Verification items for this drawing (mm, ordinates from the low corner). A direction names the side the tool comes from. Round coordinates to 2 decimals unless told otherwise and drop trailing zeros. Order: outer loops, then holes, each group sorted by start corner. A loop starts at its lowest first (then second) coordinate and runs counter-clockwise, first axis right, second up. Notation, with made-up numbers: (78, 59.5) -> (86, 59.5) arc R22 ccw to (86, 87.5) -> close; hole circle Ø10 at (2, 61). An arc over 180 degrees is marked (long way). Put each result on its own line as item: value.
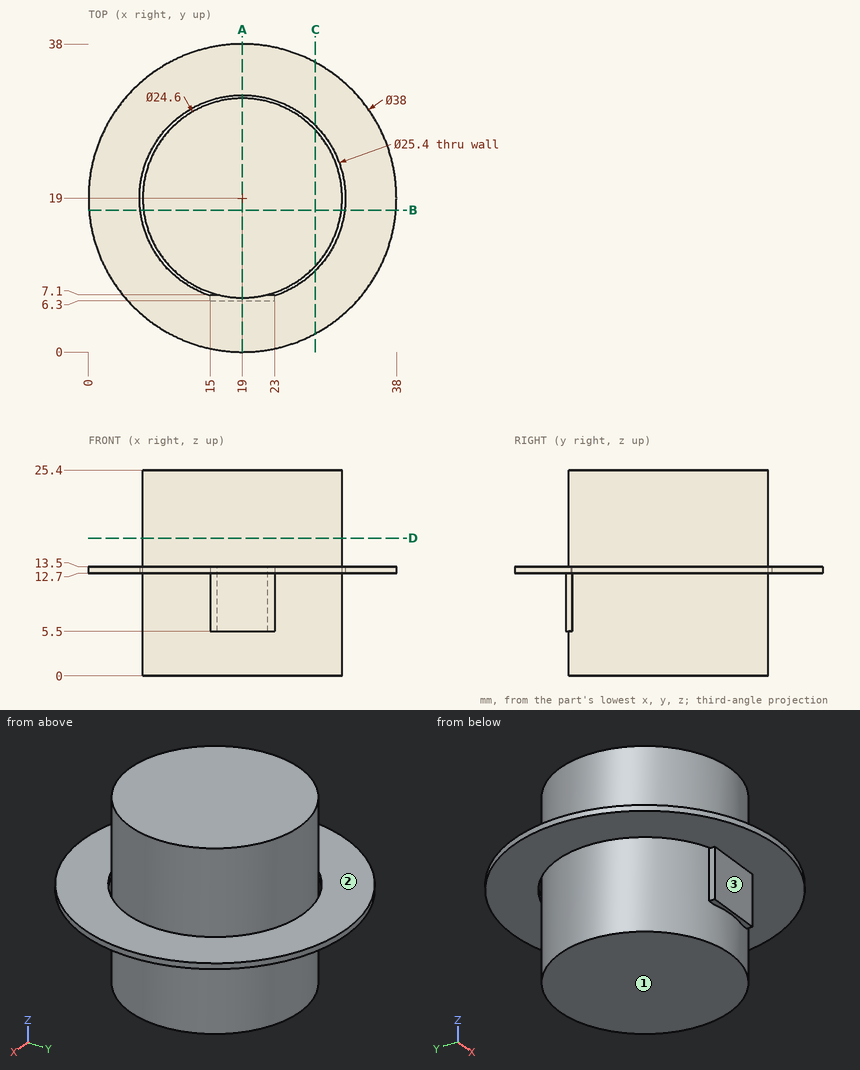
Item 1: Section check D-D on z = 17. Record the boundary of the cut face in (x, y), then the cut area to 3 significant figures.
Check sheet entries:
outline: circle Ø24.6 at (19, 19)
area: 475 mm^2
Item 2: Tool access check on the marked faces 1, 2 and 3. Record the directions out of +Z, -Z, +X, -X, +Y, -Y that give a thin tool (end or side, any length) a straight path to the whole face; none if there is none.
Check sheet entries:
face 1: -Z, +X, -X, +Y, -Y
face 2: +Z
face 3: -Z, +X, -X, -Y
Item 3: Gauge pin test, flat ends, axial feed: pin 1 Ø2 at (x, z) = (11.5, 13) entering from -Y; pin 2 Ø1.5 at (x, z) = (24.5, 22) entering from -Y; pin 3 Ø1.5 at (y, z) = (10.5, 17) entering from -X. Record the tip position at first contact, or that the pin passes through.
Check sheet entries:
pin 1: stops at y = 1.15
pin 2: stops at y = 7.65
pin 3: stops at x = 9.45
Item 4: Section check C-C on x = 28. Record the boundary of the cut face in (y, z), then the cut area to 3 significant figures.
Check sheet entries:
outline: (2.27, 12.7) -> (10.04, 12.7) -> (10.04, 13.5) -> (2.27, 13.5) -> close; (10.62, 0) -> (27.38, 0) -> (27.38, 25.4) -> (10.62, 25.4) -> close; (27.96, 12.7) -> (35.73, 12.7) -> (35.73, 13.5) -> (27.96, 13.5) -> close
area: 438 mm^2
Item 5: Section check A-A on x = 19. Record the boundary of the cut face in (y, z).
Check sheet entries:
outline: (0, 12.7) -> (6.3, 12.7) -> (6.3, 5.5) -> (6.7, 5.5) -> (6.7, 0) -> (31.3, 0) -> (31.3, 25.4) -> (6.7, 25.4) -> (6.7, 13.5) -> (0, 13.5) -> close; (31.7, 12.7) -> (38, 12.7) -> (38, 13.5) -> (31.7, 13.5) -> close
Item 6: Section check B-B on y = 17.5. Record the boundary of the cut face in (x, z).
Check sheet entries:
outline: (0.06, 12.7) -> (6.39, 12.7) -> (6.39, 13.5) -> (0.06, 13.5) -> close; (6.79, 0) -> (31.21, 0) -> (31.21, 25.4) -> (6.79, 25.4) -> close; (31.61, 12.7) -> (37.94, 12.7) -> (37.94, 13.5) -> (31.61, 13.5) -> close
Item 7: Material ranges on L1, parallel to Y at x = 19, z = 13.35; L2, parallel to X at y = 18.5, z = 7.5; L3, parallel to Z at x = 28.5, y = 7, recorded low to high. Write a range as [from, to].
Check sheet entries:
L1: y = [0, 31.3], [31.7, 38]
L2: x = [6.71, 31.29]
L3: z = [12.7, 13.5]
